Source: CAD feature listing. Evaluate the final solid. Frame: model axes, mm. Face numbers are marked on the shaded views. A direction names the side the tool comes from. Round coordinates to 2 decimals unless told otherwise and drop trailing zeros. Order: outer loops, then holes, each group sorted by start corner. A loop starts at its lowest first (then second) coordinate and runs counter-clockwise, first axis right, second up. Notation, with made-up numbers: (40, 43) -> (90, 43) arc R17 cw to (90, 75) -> close; hole circle Ø7 at (13, 70). An arc over 180 degrees is marked (long way). Answer as CSV lines item,"result".
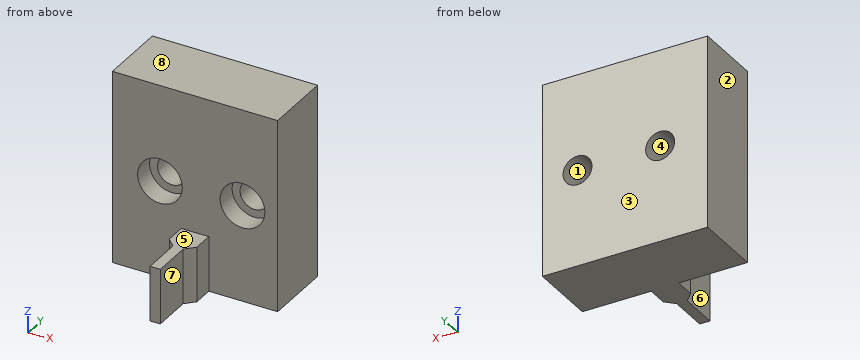
from build123d import *

# Parameters (mm, degrees)
F0_W        = 24
F0_H        = 28
F0_R        = 2.1
F1_DEPTH    = 10
F2_W        = 4
F2_H        = 8
F3_DEPTH    = 5
F4_W        = 1.5
F4_H        = 8
F5_DEPTH    = 5
F6_T4_DEPTH = 18.2867319519
F6_T9_DEPTH = 18.2867319519
F7_R        = 3.25
F8_DEPTH    = 3


# Not quite as in the source:
# - a fillet or chamfer that OpenCascade refuses, or shapes differently, is made with other operations: its cross-section is extruded or revolved along the edge and cut away or added


with BuildPart() as f1:
    # F0 (on Front) → F1 (new body)
    with BuildSketch(Plane.XZ):
        Rectangle(F0_W, F0_H)
        with Locations((-5.1, 0)):
            Circle(F0_R, mode=Mode.SUBTRACT)
        with Locations((6.9, 0)):
            Circle(F0_R, mode=Mode.SUBTRACT)
    extrude(amount=F1_DEPTH)

    # F2 (on face) → F3 (join)
    with BuildSketch(Plane.XZ.offset(10)):
        with Locations((0, -10)):
            Rectangle(F2_W, F2_H)
    extrude(amount=F3_DEPTH)

    # F4 (on face) → F5 (join)
    with BuildSketch(Plane.XZ.offset(15)):
        with Locations((0, -10)):
            Rectangle(F4_W, F4_H)
    extrude(amount=F5_DEPTH)

    # F6: chamfer of 2 on 2 edges, made by hand


with BuildPart() as f6_tool2:
    # F6_s3 → F6_t4 (new body)
    with BuildSketch(Plane.XY.offset(-19.1433659759)):
        Polygon((0, -15), (2, -13), (2, -15), align=None)
    extrude(amount=F6_T4_DEPTH)

    split(bisect_by=Plane.YZ.offset(0.75), keep=Keep.TOP)


with BuildPart() as f1_1:
    add(f1.part)

    # F6_t1: cut F6_tool2
    add(f6_tool2.part, mode=Mode.SUBTRACT)


with BuildPart() as f6_tool7:
    # F6_s8 → F6_t9 (new body)
    with BuildSketch(Plane.XY.offset(-0.8566340241)):
        Polygon((-2, -13), (0, -15), (-2, -15), align=None)
    extrude(amount=-F6_T9_DEPTH)

    split(bisect_by=Plane.YZ.offset(-0.75), keep=Keep.BOTTOM)


with BuildPart() as f1_2:
    add(f1_1.part)

    # F6_t6: cut F6_tool7
    add(f6_tool7.part, mode=Mode.SUBTRACT)

    # F7 (on face) → F8 (cut)
    with BuildSketch(Plane.XZ.offset(10)):
        with Locations((-5.1, 0)):
            Circle(F7_R)
        with Locations((6.9, 0)):
            Circle(F7_R)
    extrude(amount=-F8_DEPTH, mode=Mode.SUBTRACT)


solid = f1_2.part
1. Pin query (flat end, axial travel): pin 1 (4.5 mm diameter, centred on y = -17, z = -9, fed in from -X); pin 2 (2 mm diameter, centred on x = -6, z = 3.5, fed in from -Y); pin 3 (2.5 mm diameter, centred on y = -11, z = -11.5, fed in from +X); pin 4 (3.5 mm diameter, centred on y = -12, z = -9, fed in from -X). Return the tip coordinate at first contact, or that it passes through.
Results below:
pin 1,"x = -0.75"
pin 2,"y = -10"
pin 3,"x = 12"
pin 4,"x = -2"
2. Section query D-D on z = -11. Return loops of the section in (x, y).
Results below:
outline,"(-12, -10) -> (-2, -10) -> (-2, -13) -> (-0.75, -14.25) -> (-0.75, -20) -> (0.75, -20) -> (0.75, -14.25) -> (2, -13) -> (2, -10) -> (12, -10) -> (12, 0) -> (-12, 0) -> close"
3. Line query: L1, parallel to X at y = -2, z = 0; L2, parallel to Z at x = 6.9, y = -2.25; L3, parallel to Z at x = 6.9, y = -9.35. Output: solid intervals per line, ascending. Write a range as [from, to].
Results below:
L1,"[-12, -7.2], [-3, 4.8], [9, 12]"
L2,"[-14, -2.1], [2.1, 14]"
L3,"[-14, -3.25], [3.25, 14]"
4. Reachability of the marked faces 5, 6, 7 and 8 from +Z, -Z, +X, -X, +Y, -Y: full face, straight path, thin tool, end or side. Return the list, or none.
Results below:
face 5,"+Z, +X, -X, -Y"
face 6,"+Z, -Z, -X, -Y"
face 7,"+Z, -Z, +X, -Y"
face 8,"+Z, +X, -X, +Y, -Y"
5. Section query A-A on x = 6.9. Return loops of the section in (y, z), and give its area (3 significant figures).
Results below:
outline,"(-10, -14) -> (0, -14) -> (0, -2.1) -> (-7, -2.1) -> (-7, -3.25) -> (-10, -3.25) -> close; (-10, 3.25) -> (-7, 3.25) -> (-7, 2.1) -> (0, 2.1) -> (0, 14) -> (-10, 14) -> close"
area,"231 mm2"
6. Mould query, pull axis X, two halves, no side actions, for the marked faces 1, 2, 3 and 4. Classes: released by +X, released by -X, zero draft, split by the parting line, or undercut.
Results below:
face 1,"undercut"
face 2,"released by -X"
face 3,"zero draft"
face 4,"undercut"
7. Section query B-B on z = -1.75. Return loops of the section in (x, y), and give its area (3 significant figures).
Results below:
outline,"(-12, -10) -> (-7.84, -10) -> (-7.84, -7) -> (-6.26, -7) -> (-6.26, 0) -> (-12, 0) -> close; (-3.94, -7) -> (-2.36, -7) -> (-2.36, -10) -> (4.16, -10) -> (4.16, -7) -> (5.74, -7) -> (5.74, 0) -> (-3.94, 0) -> close; (8.06, -7) -> (9.64, -7) -> (9.64, -10) -> (12, -10) -> (12, 0) -> (8.06, 0) -> close"
area,"175 mm2"
8. Section query C-C on y = -7.75. Return loops of the section in (x, z).
Results below:
outline,"(-12, -14) -> (12, -14) -> (12, 14) -> (-12, 14) -> close; hole circle Ø6.5 at (-5.1, 0); hole circle Ø6.5 at (6.9, 0)"
